Autodesk Inventor part; units mm, degrees
ref_plane "YZ Plane" through (0, 0, 0) normal (1, 0, 0) x (0, 1, 0)
ref_plane "XZ Plane" through (0, 0, 0) normal (0, 1, 0) x (-1, 0, 0)
ref_plane "XY Plane" through (0, 0, 0) normal (0, 0, 1) x (1, 0, 0)
sketch "ExtrusionBacker_X_350mm" plane through (0, 0, 0) normal (0, 0, 1) x (1, 0, 0)
  arc A0 (340.9999, 24.106) -> (342.9999, 26.106) centre (340.9999, 26.106) ccw
  line L0 (342.9999, 26.106) -> (342.9999, 40.106)
  arc A1 (342.9999, 40.106) -> (340.9999, 42.106) centre (340.9999, 40.106) ccw
  line L1 (340.9999, 42.106) -> (-15.0001, 42.106)
  arc A2 (-15.0001, 42.106) -> (-17.0001, 40.106) centre (-15.0001, 40.106) ccw
  line L2 (-17.0001, 40.106) -> (-17.0001, 26.106)
  arc A3 (-17.0001, 26.106) -> (-15.0001, 24.106) centre (-15.0001, 26.106) ccw
  line L3 (-15.0001, 24.106) -> (340.9999, 24.106)
  line L4 (302.2499, 37.0031) -> (307.986, 33.6914)
  line L5 (307.986, 33.6914) -> (307.986, 36.2894)
  line L6 (307.986, 36.2894) -> (302.2499, 39.6012)
  line L7 (302.2499, 39.6012) -> (302.2499, 37.0031)
  line L8 (296.5137, 37.7168) -> (296.5137, 35.1187)
  line L9 (296.5137, 35.1187) -> (307.986, 28.4952)
  line L10 (307.986, 28.4952) -> (307.986, 31.0933)
  line L11 (307.986, 31.0933) -> (296.5137, 37.7168)
  line L12 (296.5137, 32.5207) -> (296.5137, 29.9226)
  line L13 (296.5137, 29.9226) -> (302.2499, 26.6108)
  line L14 (302.2499, 26.6108) -> (302.2499, 29.2089)
  line L15 (302.2499, 29.2089) -> (296.5137, 32.5207)
  circle A4 centre (122.9999, 33.106) radius 1.7
  circle A5 centre (202.9999, 33.106) radius 1.7
  circle A6 centre (242.9999, 33.106) radius 1.7
  circle A7 centre (162.9999, 33.106) radius 1.7
  circle A8 centre (3.9999, 38.106) radius 1
  circle A9 centre (3.9999, 28.106) radius 1
  circle A10 centre (11.9999, 33.106) radius 1
  circle A11 centre (42.9999, 33.106) radius 1.7
  circle A12 centre (82.9999, 33.106) radius 1.7
  circle A13 centre (282.9999, 33.106) radius 1.7
  circle A14 centre (19.9999, 33.106) radius 1
  circle A15 centre (2.9999, 33.106) radius 1.7
  circle A16 centre (322.9999, 33.106) radius 1.7
  circle A17 centre (7.9999, 33.106) radius 1
sketch "Skizze1" plane through (0, 0, 0) normal (0, 1, 0) x (-1, 0, 0)
  arc A0 (338, -9) -> (340, -7) centre (338, -7) ccw
  line L0 (340, -7) -> (340, 7)
  arc A1 (340, 7) -> (338, 9) centre (338, 7) ccw
  line L1 (338, 9) -> (-18, 9)
  arc A2 (-18, 9) -> (-20, 7) centre (-18, 7) ccw
  line L2 (-20, 7) -> (-20, -7)
  arc A3 (-20, -7) -> (-18, -9) centre (-18, -7) ccw
  line L3 (-18, -9) -> (338, -9)
  line L4 (299.25, 3.8971) -> (304.9862, 0.5853)
  line L5 (304.9862, 0.5853) -> (304.9862, 3.1834)
  line L6 (304.9862, 3.1834) -> (299.25, 6.4952)
  line L7 (299.25, 6.4952) -> (299.25, 3.8971)
  line L8 (293.5138, 4.6108) -> (293.5138, 2.0127)
  line L9 (293.5138, 2.0127) -> (304.9862, -4.6108)
  line L10 (304.9862, -4.6108) -> (304.9862, -2.0127)
  line L11 (304.9862, -2.0127) -> (293.5138, 4.6108)
  line L12 (293.5138, -0.5853) -> (293.5138, -3.1834)
  line L13 (293.5138, -3.1834) -> (299.25, -6.4952)
  line L14 (299.25, -6.4952) -> (299.25, -3.8971)
  line L15 (299.25, -3.8971) -> (293.5138, -0.5853)
  circle A4 centre (120, 0) radius 1.7
  circle A5 centre (200, 0) radius 1.7
  circle A6 centre (240, 0) radius 1.7
  circle A7 centre (160, 0) radius 1.7
  circle A8 centre (1, 5) radius 1
  circle A9 centre (1, -5) radius 1
  circle A10 centre (9, 0) radius 1
  circle A11 centre (40, 0) radius 1.7
  circle A12 centre (80, 0) radius 1.7
  circle A13 centre (280, 0) radius 1.7
  circle A14 centre (17, 0) radius 1
  circle A15 centre (0, 0) radius 1.7
  circle A16 centre (320, 0) radius 1.7
  circle A17 centre (5, 0) radius 1
  point P0 (338, -9)
  point P1 (340, 7)
  point P2 (338, 9)
  point P3 (-18, 9)
  point P4 (-20, 7)
  point P5 (-20, -7)
  point P6 (-18, -9)
  point P7 (293.5138, -0.5853)
  point P8 (299.25, -3.8971)
  point P9 (299.25, -6.4952)
  point P10 (293.5138, -3.1834)
  point P11 (293.5138, 4.6108)
  point P12 (304.9862, -2.0127)
  point P13 (304.9862, -4.6108)
  point P14 (293.5138, 2.0127)
  point P15 (299.25, 3.8971)
  point P16 (299.25, 6.4952)
  point P17 (304.9862, 3.1834)
  point P18 (304.9862, 0.5853)
extrude "Extrusion1" add sketch "Skizze1" along normal blind 2
sketch "Skizze2" plane through (0, 2, 0) normal (0, 1, 0) x (1, 0, 0)
  circle A0 centre (-320, 0) radius 1.7
  circle A1 centre (-280, 0) radius 1.7
  circle A2 centre (-240, 0) radius 1.7
  circle A3 centre (-200, 0) radius 1.7
  circle A4 centre (-160, 0) radius 1.7
  circle A5 centre (-120, 0) radius 1.7
  circle A6 centre (-80, 0) radius 1.7
  circle A7 centre (-40, 0) radius 1.7
  circle A8 centre (0, 0) radius 1.7
  point P0 (-81.3289, 1.9857)
hole "Bohrung1" at (-320, 2, 0) at (-280, 2, 0) at (-240, 2, 0) at (-200, 2, 0) at (-160, 2, 0) at (-120, 2, 0) at (-80, 2, 0) at (-40, 2, 0) at (0, 2, 0) direction (0, -1, 0) diameter 3.4 end through all countersink diameter 7.5 countersink angle 90
properties part number "X Extrusion-Backer (350mm)" material "Titan"
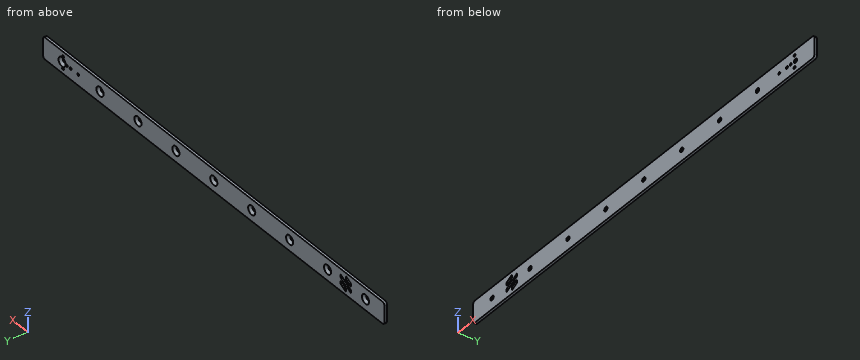
Input: part model. Units: mm. Frame: model coordinates. Coordinates: 2 decimals unless noted, no trailing zeros. Order: outer loops, then holes, each group sorted by start corner. A loop starts at its lowest first (then second) coordinate and runs counter-clockwise, first axis right, second up. Notation, with made-up numbers: M 82,-7.75 L 87,-7.75 A12 ccw 87,11.25 Z; hole C 81,-10 d11. An arc over 180 degrees is marked long. Write item = value, one per line. Start each with the question number.
(1) Section A-A on y = 0.9. Give the number of separate pieces and of enclosed holes in the cut face, and give its area (3 significant figures).
(2) First-contact query: P1, Ø1.6, axis at x = -17, z = 0, coming from the +Y side. Flat tip, straight axial feed; report the tip coordinate or a pass-through.
(3) Line query: line 1 along Z through (x, y) = (-1, 1.6); line 2 along Z through (x, y) = (-17, 1); line 3 along X through (y, z) = (1.35, 5.75). Output: solid intervals per line, ascending. Write a range as [from, to].
(4) Section B-B on x = -320. Output: boundary loops of the cut face in (y, z), and give its area (3 significant figures).
Result set:
q1.separate_pieces = 1
q1.enclosed_holes = 17
q1.area = 6,200 mm²
q2.P1 = through
q3.line_1 = [-9, -6], [-4, -3.2], [3.2, 4], [6, 9]
q3.line_2 = [-9, -1], [1, 9]
q3.line_3 = [-340, -300.54], [-299.25, -1.66], [-0.34, 20]
q4.outline = M 0,-9 L 2,-9 L 2,-3.75 L 0,-1.75 Z; M 0,1.75 L 2,3.75 L 2,9 L 0,9 Z
q4.area = 25.0 mm²
